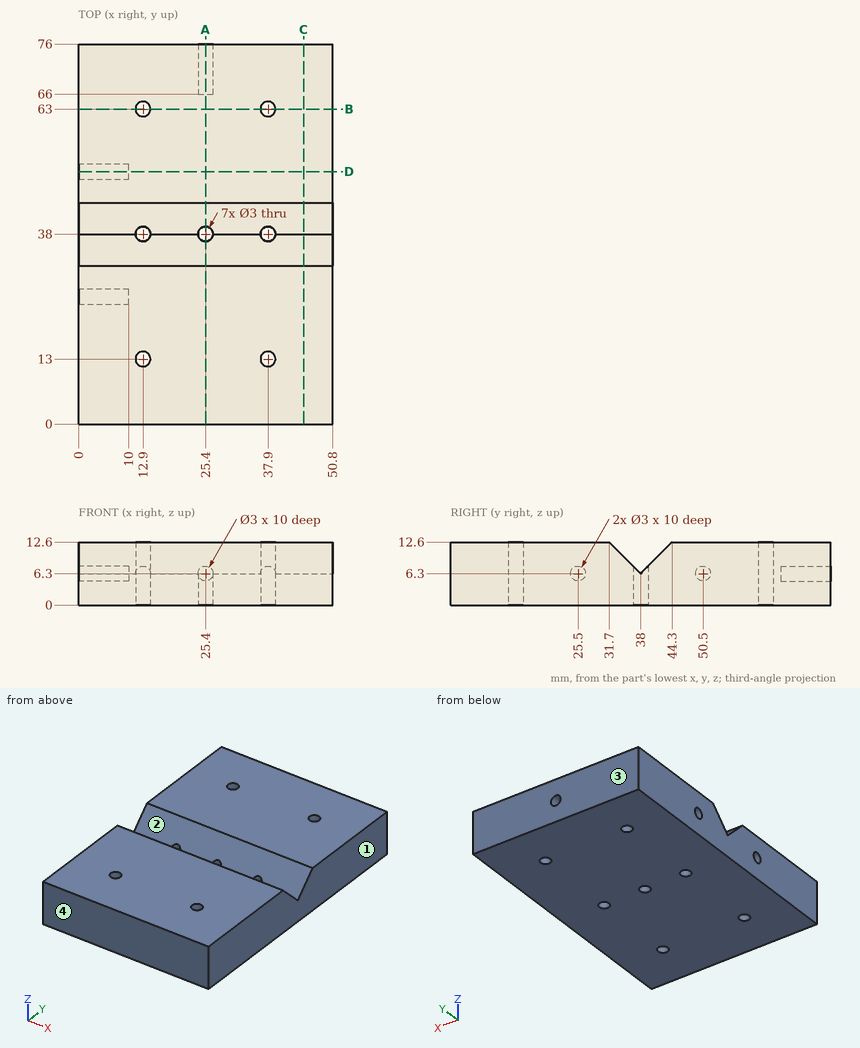
Print and shaded views of the part. All mm, measured from the part's lowest x, y and z. Round coordinates to 2 decimals unless told otherwise and drop trailing zeros. Write each loop counter-clockwise with the first axis right and the second up, starting at its lowest first coordinate (ties: lowest second). Pieces come first, ordered by that corner, then holes. Notation, with made-up numbers: (86.5, 70.5) - (106.5, 70.5) arc R6 ccw to (106.5, 74.5) - close; hole circle Ø2 at (42.25, 0). An arc over 180 degrees is marked (long way). Write each question's results on one line, items separated by ' | '. Start each with the question number.
Item 1: Mould opens along Y. For the marked faces 1, 2, 3 and 4 say: pulls with the +Y half, pulls with the -Y half, needs draft (parallel to the pull), parting line crosses it, or undercut.
Item 2: Saw through at B-B (y = 63). Write the cut outline in (x, z), and give its area (3 significant figures).
Item 3: Saw through at C-C (x = 45). Write the cut outline in (y, z).
Item 4: Saw through at D-D (y = 50.5). Write the cut outline in (x, z), and give its area (3 significant figures).
Item 5: Drop flat-ended pins along their axis: P1, Ø2.5, axis at x = 12.9, y = 13, coming from the +Z side; P2, Ø4, axis at x = 37.9, y = 38, coming from the +Z side; P3, Ø2.5, axis at y = 25.5, z = 6.3, coming from the -X side. Give the stop position or say it passes through.
Item 6: Wall check: L1, parallel to Y at x = 12.9, z = 6; L2, parallel to X at y = 38, z = 5.5; L3, parallel to Y at x = 6.5, z = 6.25. Give the ranges that are in metal, low to high. Write a range as [from, to].
Item 7: Saw through at A-A (x = 25.4). Write the cut outline in (y, z), and give its area (3 significant figures).
Results are:
1) face 1: needs draft | face 2: undercut | face 3: pulls with the +Y half | face 4: pulls with the -Y half
2) outline: (0, 0) - (11.4, 0) - (11.4, 12.6) - (0, 12.6) - close; (14.4, 0) - (36.4, 0) - (36.4, 12.6) - (14.4, 12.6) - close; (39.4, 0) - (50.8, 0) - (50.8, 12.6) - (39.4, 12.6) - close | area: 564 mm²
3) outline: (0, 0) - (76, 0) - (76, 12.6) - (44.3, 12.6) - (38, 6.3) - (31.7, 12.6) - (0, 12.6) - close
4) outline: (0, 0) - (50.8, 0) - (50.8, 12.6) - (0, 12.6) - (0, 7.8) - (10, 7.8) - (10, 4.8) - (0, 4.8) - close | area: 610 mm²
5) P1: passes through | P2: stops at z = 8.3 | P3: stops at x = 10
6) L1: y = [0, 11.5], [14.5, 36.5], [39.5, 61.5], [64.5, 76] | L2: x = [0, 11.4], [14.4, 23.9], [26.9, 36.4], [39.4, 50.8] | L3: y = [0, 24], [27, 49], [52, 76]
7) outline: (0, 0) - (36.5, 0) - (36.5, 7.8) - (31.7, 12.6) - (0, 12.6) - close; (39.5, 0) - (76, 0) - (76, 4.8) - (66, 4.8) - (66, 7.8) - (76, 7.8) - (76, 12.6) - (44.3, 12.6) - (39.5, 7.8) - close | area: 867 mm²
